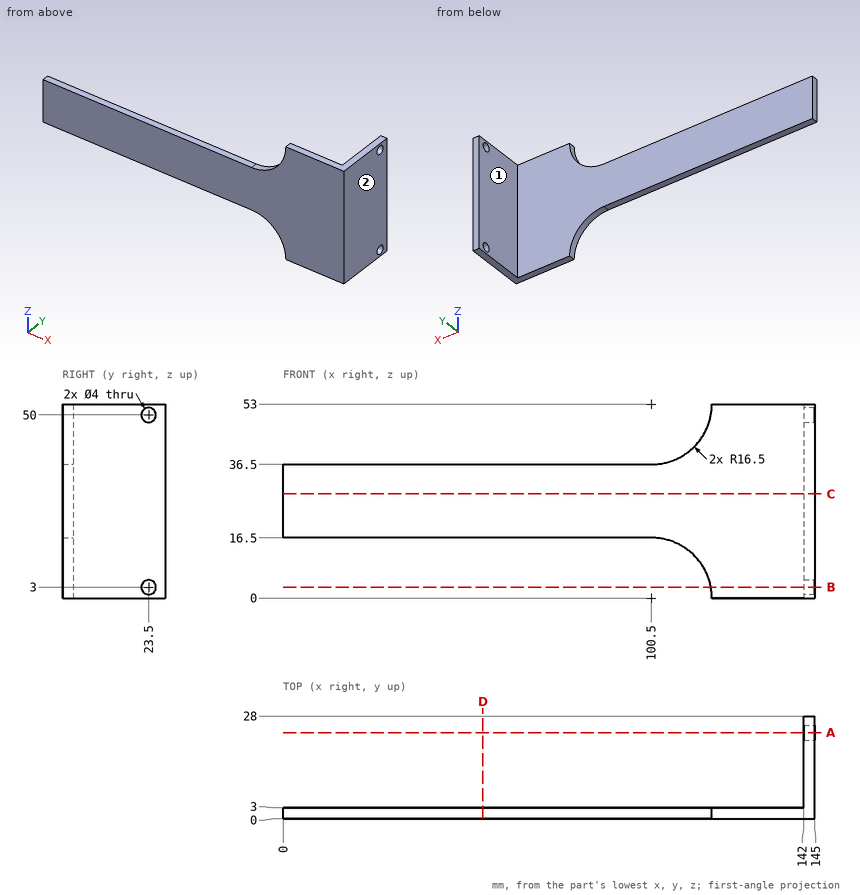
Could you check a few things on this drawing? It's one solid part, dimensions in mm from its lowest x, y, z. A direction names the side the tool comes from. Coordinates: 2 decimals unless noted, no trailing zeros. Loops run counter-clockwise (first coordinate to the right, second up) from the corner with the lowest first, then second, coordinate; pieces in that order, holes last.
1. Imagine slicing it at C-C (z = 28.5). Please give me the cut outline in (x, y), and give its area (3 significant figures).
2. Imagine slicing it at A-A (y = 23.5). Please give me the cut outline in (x, z).
3. Imagine slicing it at B-B (z = 3). Please give me the cut outline in (x, y).
4. For P1, Ø5, axis at y = 23.5, z = 50, coming from the -X side; P2, Ø0.9, axis at x = 70, y = 1, coming from the -Z side; P3, Ø3, axis at y = 23.5, z = 3, coming from the +X side; P4, Ø6, axis at x = 24, z = 25.5, coming from the +Y side, each with a flat end and sliding along its axis, tell me the tip position at first contact or that it passes through.
5. For the marked faces 1 and 2, which set-ups out of +Z, -Z, +X, -X, +Y, -Y let a thin tool reach every point of the face, with its end or its side?
6. Imagine slicing it at D-D (x = 54.5). Please give me the cut outline in (y, z).
7. I need wall thicknesses on L1, parallel to Y at x = 143, z = 50; L2, parallel to X at y = 13.25, z = 49; L3, parallel to Y at x = 136, z = 47.5. Which ranges of each line are inside material? Lowest first, please.
Computed values:
1. outline: (0, 0) - (145, 0) - (145, 28) - (142, 28) - (142, 3) - (0, 3) - close
1. area: 510 mm2
2. outline: (142, 0) - (145, 0) - (145, 1) - (142, 1) - close; (142, 5) - (145, 5) - (145, 48) - (142, 48) - close; (142, 52) - (145, 52) - (145, 53) - (142, 53) - close
3. outline: (116.72, 0) - (145, 0) - (145, 21.5) - (142, 21.5) - (142, 3) - (116.72, 3) - close; (142, 25.5) - (145, 25.5) - (145, 28) - (142, 28) - close
4. P1: stops at x = 142
4. P2: stops at z = 16.5
4. P3: passes through
4. P4: stops at y = 3
5. face 1: +Z, -Z, -X, +Y
5. face 2: +Z, -Z, +X, +Y, -Y
6. outline: (0, 16.5) - (3, 16.5) - (3, 36.5) - (0, 36.5) - close
7. L1: y = 0 to 21.5, 25.5 to 28
7. L2: x = 142 to 145
7. L3: y = 0 to 3
